Autodesk Inventor part; units mm, degrees
ref_plane "YZ Plane" through (0, 0, 0) normal (1, 0, 0) x (0, 1, 0)
ref_plane "XZ Plane" through (0, 0, 0) normal (0, 1, 0) x (-1, 0, 0)
ref_plane "XY Plane" through (0, 0, 0) normal (0, 0, 1) x (1, 0, 0)
ref_plane "작업 평면1" through (23.5, -8, -2) normal (1, 0, 0) x (0, 0, -1)
sketch "스케치1" plane through (23.5, -8, -2) normal (1, 0, 0) x (0, 0, -1)
  line L0 (0, 16) -> (-8.15, 16)
  line L1 (-8.15, 16) -> (-8.15, 10.6)
  line L2 (-8.15, 10.6) -> (-12.15, 10.6)
  line L3 (-13.15, 9.6) -> (-12.15, 10.6)
  line L4 (-13.15, 9.6) -> (-13.15, 6.4)
  line L5 (-12.15, 5.4) -> (-13.15, 6.4)
  line L6 (-12.15, 5.4) -> (-8.15, 5.4)
  line L7 (-8.15, 5.4) -> (-8.15, 0)
  line L8 (-8.15, 0) -> (0, 0)
  line L9 (0, 16) -> (6.35, 16)
  line L10 (6.35, 16) -> (6.35, 15)
  line L11 (6.35, 15) -> (5.35, 14)
  line L12 (4.35, 14) -> (4.35, 2)
  line L13 (4.35, 14) -> (5.35, 14)
  line L14 (0, 0) -> (6.35, 0)
  line L15 (6.35, 0) -> (6.35, 1)
  line L16 (6.35, 1) -> (5.35, 2)
  line L17 (4.35, 2) -> (5.35, 2)
  line L18 (0, 16) -> (-8.15, 16)
  line L19 (-8.15, 10.6) -> (-12.15, 10.6)
  line L20 (-8.15, 10.6) -> (-12.15, 10.6)
  line L21 (-12.15, 10.6) -> (-13.15, 9.6)
  line L22 (-13.15, 6.4) -> (-12.15, 5.4)
  point P0 (-2, 8)
  dimension "d1" = 6.35
sketch "스케치2" plane through (-23.5, 8, 6.15) normal (0, 0, 1) x (1, 0, 0)
  arc A0 (7.9209, -9.6) -> (7.9209, -6.4) centre (6, -8) ccw
  line L0 (39.0791, -9.6) -> (7.9209, -9.6)
  circle A1 centre (6, -8) radius 2.5
  circle A2 centre (41, -8) radius 2.5
  circle A3 centre (41, -8) radius 2.5
  point P0 (23.5, -8)
  point P1 (7.9209, -6.4)
extrude "돌출1" add sketch "스케치1" against normal up to surface (47 mm away)
extrude "돌출2" cut sketch "스케치2" along normal mid plane 50
sketch "스케치3" plane through (-15.5791, 1.6, 11.15) normal (0, 0, 1) x (1, 0, 0)
  line L0 (15.5791, -14.4593) -> (15.5791, 15.5737)
  line L1 (-7.9209, 4.4) -> (-7.9209, -7.6)
  line L2 (-7.9209, 4.4) -> (11.0791, 4.4)
  line L3 (11.0791, 4.4) -> (11.0791, -7.6)
  line L4 (11.0791, -7.6) -> (-7.9209, -7.6)
  line L5 (-7.9209, -7.6) -> (-7.9209, 4.4)
  line L6 (39.0791, 4.4) -> (39.0791, -7.6)
  line L7 (39.0791, 4.4) -> (20.0791, 4.4)
  line L8 (20.0791, 4.4) -> (20.0791, -7.6)
  line L9 (20.0791, -7.6) -> (39.0791, -7.6)
  line L10 (39.0791, -7.6) -> (39.0791, 4.4)
  point P0 (15.5791, -1.6)
  dimension "d9" = 19
extrude "돌출3" cut sketch "스케치3" against normal up to surface (5 mm away)
sketch "스케치4" plane through (-23.5, 8, 6.15) normal (0, 0, 1) x (1, 0, 0)
  circle A0 centre (6, -8) radius 2.5
  circle A1 centre (6, -8) radius 3
  circle A2 centre (41, -8) radius 2.5
  circle A3 centre (41, -8) radius 3
  point P0 (23.5, -8)
  dimension "d10" = 6
  dimension "d11" = 6
extrude "돌출4" cut sketch "스케치4" against normal up to surface (12.5 mm away) contours A0 | A1 | A2 | A3
properties part number "Bearing Spacer"
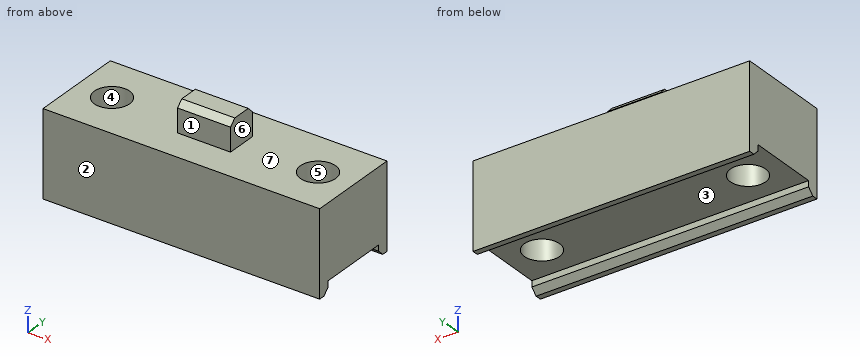
Check sheet for the modelled part. Datum: model origin and axes. Units: mm. Face numbers are marked on the shaded views. A direction names the side the tool comes from. Round coordinates to 2 decimals unless told otherwise and drop trailing zeros. Loops run counter-clockwise (first coordinate to the right, second up) from the corner with the lowest first, then second, coordinate; pieces in that order, holes last. Notation, with made-up numbers: M -0.5,-19.75 L 43.5,-19.75 A28 ccw 43.5,16.25 Z; hole C 86,56.5 d8. An arc over 180 degrees is marked long. One line per item, written item: value.
(1) Depth check by flat-ended pin: pin 1 Ø6 at (x, y) = (-15.5, -1) entering from +Z; pin 2 Ø1.5 at (y, z) = (-0.5, 7.5) entering from +X; pin 3 Ø3.5 at (x, y) = (-6.5, 2.5) entering from -Z. Enter the tip coordinate at first touch or a pass-through.
Computed values:
pin 1: stops at z = 6.15
pin 2: stops at x = 4.5
pin 3: stops at z = -6.35
(2) Sectioned sample at A-A, the plane x = 17.5. Record the cut outline in (y, z), then the cut area to 3 significant figures.
Computed values:
outline: M -8,-8.35 L -7,-8.35 L -6,-7.35 L -6,-6.35 L -3,-6.35 L -3,6.15 L -8,6.15 Z; M 3,-6.35 L 6,-6.35 L 6,-7.35 L 7,-8.35 L 8,-8.35 L 8,6.15 L 3,6.15 Z
area: 132 mm^2
(3) Sectioned sample at C-C, the plane x = -1.5. Record the cut outline in (y, z).
Computed values:
outline: M -8,-8.35 L -7,-8.35 L -6,-7.35 L -6,-6.35 L 6,-6.35 L 6,-7.35 L 7,-8.35 L 8,-8.35 L 8,6.15 L 2.6,6.15 L 2.6,10.15 L 1.6,11.15 L -1.6,11.15 L -2.6,10.15 L -2.6,6.15 L -8,6.15 Z
(4) Sectioned sample at B-B, the plane y = 0. Record the cut outline in (x, z), then the cut area to 4 significant figures.
Computed values:
outline: M -23.5,-6.35 L -20.5,-6.35 L -20.5,6.15 L -23.5,6.15 Z; M -14.5,-6.35 L 14.5,-6.35 L 14.5,6.15 L 4.5,6.15 L 4.5,11.15 L -4.5,11.15 L -4.5,6.15 L -14.5,6.15 Z; M 20.5,-6.35 L 23.5,-6.35 L 23.5,6.15 L 20.5,6.15 Z
area: 482.5 mm^2
(5) Release check for a two-part mould opening along X. For the marked faces 4, 5, 6 and 7 record: +X half, -X half, draft (parallel to the pull), parting line (faces both ways), or undercut.
Computed values:
face 4: undercut
face 5: undercut
face 6: +X half
face 7: draft
(6) Sectioned sample at D-D, the plane z = 1.5. Record the cut outline in (x, y), then the cut area to 3 significant figures.
Computed values:
outline: M -23.5,-8 L 23.5,-8 L 23.5,8 L -23.5,8 Z; hole C -17.5,0 d6; hole C 17.5,0 d6
area: 695 mm^2
(7) Access from +Z, -Z, +X, -X, +Y, -Y to the whole of each face (thin tool, end or side, straight path). Record for the marked faces 1, 2 and 3.
Computed values:
face 1: +Z, +X, -X, -Y
face 2: +Z, -Z, +X, -X, -Y
face 3: -Z, +X, -X
(8) Thickness scan on line 1 (X direction, y = 2.5, z = -3.5); line 2 (X direction, y = 1.5, z = -5); line 3 (Y direction, x = -17.5, z = 0.75). Record the ranges inside material, lowest first.
Computed values:
line 1: x = -23.5 to -19.16, -15.84 to 15.84, 19.16 to 23.5
line 2: x = -23.5 to -20.1, -14.9 to 14.9, 20.1 to 23.5
line 3: y = -8 to -3, 3 to 8
